from build123d import *

# Parameters (mm, degrees)
SKIZZE1_R                       = 2.54
AUFSATZ_LINEAR_AUSTRAGEN1_DEPTH = 5


with BuildPart() as part:
    # Skizze1 → Aufsatz-Linear austragen1 (new body)
    with BuildSketch(Plane.XY):
        with BuildLine():
            Line((9.866806535, -39.166387358), (26.373711346, -39.166387358))
            add(Edge.make_bspline(
                [(26.373711346, -39.166387358), (28.913711346, -39.166387358), (28.913711346, -36.622901599)],
                knots=[3.141592654, 3.141592654, 3.141592654, 4.71238898, 4.71238898, 4.71238898], degree=2, weights=[1, 0.707106781, 1]))
            Line((28.913711346, -36.622901599), (28.913711346, 36.821129628))
            ThreePointArc((28.913711346, 36.821129628), (28.169762571, 38.617180852), (26.373711346, 39.361129628))
            Line((26.373711346, 39.361129628), (-24.426288654, 39.361129628))
            ThreePointArc((-24.426288654, 39.361129628), (-26.222339878, 38.617180852), (-26.966288654, 36.821129628))
            Line((-26.966288654, 36.821129628), (-26.966288654, -36.622901599))
            add(Edge.make_bspline(
                [(-26.966288654, -36.622901599), (-26.966288654, -39.166387358), (-24.426288654, -39.166387358)],
                knots=[1.570796327, 1.570796327, 1.570796327, 3.141592654, 3.141592654, 3.141592654], degree=2, weights=[1, 0.707106781, 1]))
            Line((-24.426288654, -39.166387358), (-7.919383842, -39.166387358))
            add(Edge.make_bspline(
                [(-7.919383842, -39.166387358), (-7.896041529, -39.166387358), (-7.872713398, -39.165529461)],
                knots=[0.586855187, 0.586855187, 0.586855187, 0.623588271, 0.623588271, 0.623588271], degree=2, weights=[1, 0.99983134, 1]))
            Line((-7.872713398, -39.165529461), (9.866806535, -39.166387358))
        make_face()
        with Locations((-19.663788654, -31.343187358)):
            Circle(SKIZZE1_R, mode=Mode.SUBTRACT)
        with Locations((21.611211346, -31.343187358)):
            Circle(SKIZZE1_R, mode=Mode.SUBTRACT)
        with Locations((21.611211346, 32.156812642)):
            Circle(SKIZZE1_R, mode=Mode.SUBTRACT)
        with Locations((21.611211346, 22.631812642)):
            Circle(SKIZZE1_R, mode=Mode.SUBTRACT)
        with Locations((-19.663788654, 22.631812642)):
            Circle(SKIZZE1_R, mode=Mode.SUBTRACT)
        with Locations((-19.663788654, 32.156812642)):
            Circle(SKIZZE1_R, mode=Mode.SUBTRACT)
    extrude(amount=AUFSATZ_LINEAR_AUSTRAGEN1_DEPTH)


solid = part.part
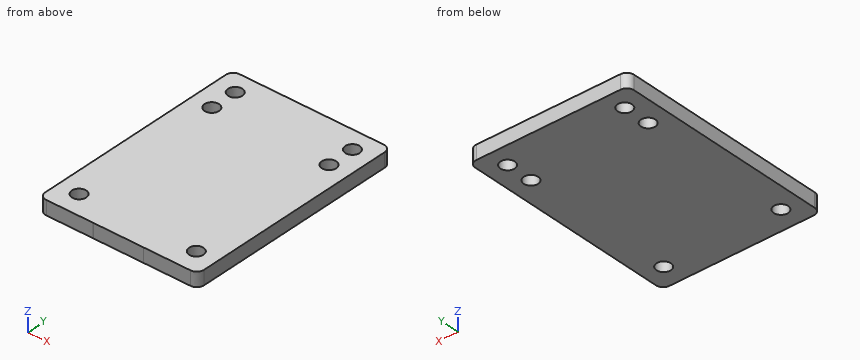
Work out the finished part from the listing and answer in its coordinate system (mm). Coordinates: 2 decimals unless noted, no trailing zeros. Order: outer loops, then holes, each group sorted by start corner. A loop starts at its lowest first (then second) coordinate and runs counter-clockwise, first axis right, second up. Notation, with made-up numbers: (86, -14.75) - (104, -14.75) arc R12 cw to (104, -3.75) - close; hole circle Ø2 at (-5.5, -30). An arc over 180 degrees is marked (long way). Put each result on its own line as item: value. Start each with the question number.
1) Find the intervals of material crossed by line 1 (X direction, y = -30, z = 4.25); line 2 (X direction, y = -29.5, z = 2.8); line 3 (Y direction, x = -24.5, z = 1.6), in increasing order. Write a range as from..to.
2) Find section C-C (z = 1.1). State how many separate pieces and enclosed holes the cut face has, plus the area to 3 significant figures.
3) Find section A-A (x = -18). Give the vertices of the cut face in (y, z).
4) Find section B-B (y = 33.5). Give the vertices of the cut face in (x, z).
Results list:
1. line 1: x = -26.97..-21.82, -17.51..19.46, 23.77..28.91
1. line 2: x = -26.97..-21.41, -17.92..19.86, 23.36..28.91
1. line 3: y = -39.17..39.36
2. separate pieces: 1
2. enclosed holes: 6
2. area: 4,260 mm^2
3. outline: (-39.17, 0) - (-33.26, 0) - (-33.26, 5) - (-39.17, 5) - close; (-29.42, 0) - (20.71, 0) - (20.71, 5) - (-29.42, 5) - close; (24.55, 0) - (30.24, 0) - (30.24, 5) - (24.55, 5) - close; (34.08, 0) - (39.36, 0) - (39.36, 5) - (34.08, 5) - close
4. outline: (-26.97, 0) - (-21.82, 0) - (-21.82, 5) - (-26.97, 5) - close; (-17.51, 0) - (19.46, 0) - (19.46, 5) - (-17.51, 5) - close; (23.77, 0) - (28.91, 0) - (28.91, 5) - (23.77, 5) - close
